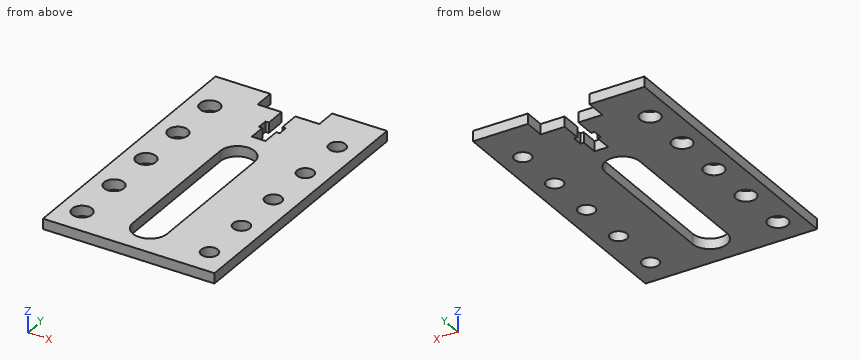
```python
from build123d import *

# Parameters (mm, degrees)
ESQUISSE1_W             = 50
ESQUISSE1_H             = 81
BOSS_EXTRU_1_DEPTH      = 3
ESQUISSE2_W             = 18
ESQUISSE2_H             = 6
ENL_V_MAT_EXTRU_1_DEPTH = 3
ENL_V_MAT_EXTRU_2_DEPTH = 3
ESQUISSE5_R             = 2.885610726
ESQUISSE5_R_2           = 2.423229835
ENL_V_MAT_EXTRU_3_DEPTH = 3


with BuildPart() as part:
    # Esquisse1 → Boss.-Extru.1 (new body)
    with BuildSketch(Plane.XY):
        with Locations((-16.166294243, 13.176556017)):
            Rectangle(ESQUISSE1_W, ESQUISSE1_H)
    extrude(amount=BOSS_EXTRU_1_DEPTH)

    # Esquisse2 → Enlèv. mat.-Extru.1 (cut)
    with BuildSketch(Plane.XY.offset(3)):
        with Locations((-16.166294243, 50.676556017)):
            Rectangle(ESQUISSE2_W, ESQUISSE2_H)
    extrude(amount=-ENL_V_MAT_EXTRU_1_DEPTH, mode=Mode.SUBTRACT)

    # Esquisse3 → Enlèv. mat.-Extru.2 (cut)
    with BuildSketch(Plane.XY.offset(3)):
        Polygon((-18.166294243, 41.676556017), (-19.166294243, 41.676556017), (-19.166294243, 38.676556017), (-18.166294243, 38.676556017), (-18.166294243, 33.676556017), (-14.166294243, 33.676556017), (-14.166294243, 38.676556017), (-13.166294243, 38.676556017), (-13.166294243, 41.676556017), (-14.166294243, 41.676556017), (-14.166294243, 47.676556017), (-18.166294243, 47.676556017), align=None)
        with BuildLine():
            Line((-11.166294243, 23.676556017), (-11.166294243, -17.323443983))
            ThreePointArc((-11.166294243, -17.323443983), (-16.166294243, -22.323443983), (-21.166294243, -17.323443983))
            Line((-21.166294243, -17.323443983), (-21.166294243, 23.676556017))
            ThreePointArc((-21.166294243, 23.676556017), (-16.166294243, 28.676556017), (-11.166294243, 23.676556017))
        make_face()
    extrude(amount=-ENL_V_MAT_EXTRU_2_DEPTH, mode=Mode.SUBTRACT)

    # Esquisse5 → Enlèv. mat.-Extru.3 (cut)
    with BuildSketch(Plane.XY.offset(3)):
        with Locations((-34.741294243, -19.323443983)):
            Circle(ESQUISSE5_R)
        with Locations((2.408705757, -19.323443983)):
            Circle(ESQUISSE5_R_2)
        with Locations((-34.741294243, -4.323443983)):
            Circle(ESQUISSE5_R)
        with Locations((2.408705757, -4.323443983)):
            Circle(ESQUISSE5_R_2)
        with Locations((-34.741294243, 10.676556017)):
            Circle(ESQUISSE5_R)
        with Locations((2.408705757, 10.676556017)):
            Circle(ESQUISSE5_R_2)
        with Locations((-34.741294243, 25.676556017)):
            Circle(ESQUISSE5_R)
        with Locations((2.408705757, 25.676556017)):
            Circle(ESQUISSE5_R_2)
        with Locations((-34.741294243, 40.676556017)):
            Circle(ESQUISSE5_R)
        with Locations((2.408705757, 40.676556017)):
            Circle(ESQUISSE5_R_2)
    extrude(amount=-ENL_V_MAT_EXTRU_3_DEPTH, mode=Mode.SUBTRACT)


solid = part.part
```
Geometry check sheet. Reference: the model listing, model coordinates, mm. Coordinates: 2 decimals unless noted, no trailing zeros. Loops run counter-clockwise (first coordinate to the right, second up) from the corner with the lowest first, then second, coordinate; pieces in that order, holes last.
Item 1: Thickness scan on line 1 (Y direction, x = -18.5, z = 0.3); line 2 (X direction, y = 2, z = 2.6); line 3 (X direction, y = 24, z = 0.3). Record the ranges inside material, lowest first.
Item 2: Sectioned sample at B-B, the plane x = -16. Record the boundary of the cut face in (y, z), then the cut area to 3 significant figures.
Item 3: Sectioned sample at C-C, the plane z = 2.1. Count the separate pieces of the cut face and the enclosed holes in it, then the cut area to 3 significant figures.
Item 4: Go/stop test with a flat-tipped pin: pin 1 Ø1.1 at (x, z) = (-13.5, 1.5) entering from +Y. Record where the tip stops, or that it passes through.
Item 5: Sectioned sample at A-A, the plane y = 5. Record the boundary of the cut face in (x, z), then the cut area to 3 significant figures.
Item 6: Sectioned sample at D-D, the plane y = -18.5. Record the boundary of the cut face in (x, z).
Check result:
1. line 1: y = -27.32 to -21.75, 28.1 to 38.68, 41.68 to 47.68
1. line 2: x = -41.17 to -21.17, -11.17 to 8.83
1. line 3: x = -41.17 to -37.09, -32.39 to -21.16, -11.18 to 0.66, 4.16 to 8.83
2. outline: (-27.32, 0) - (-22.32, 0) - (-22.32, 3) - (-27.32, 3) - close; (28.67, 0) - (33.68, 0) - (33.68, 3) - (28.67, 3) - close
2. area: 30.0 mm2
3. separate pieces: 1
3. enclosed holes: 11
3. area: 3,170 mm2
4. pin 1: stops at y = 47.68
5. outline: (-41.17, 0) - (-21.17, 0) - (-21.17, 3) - (-41.17, 3) - close; (-11.17, 0) - (8.83, 0) - (8.83, 3) - (-11.17, 3) - close
5. area: 120 mm2
6. outline: (-41.17, 0) - (-37.51, 0) - (-37.51, 3) - (-41.17, 3) - close; (-31.98, 0) - (-21.03, 0) - (-21.03, 3) - (-31.98, 3) - close; (-11.31, 0) - (0.13, 0) - (0.13, 3) - (-11.31, 3) - close; (4.69, 0) - (8.83, 0) - (8.83, 3) - (4.69, 3) - close
